from build123d import *

# Parameters (mm, degrees)
F1_DEPTH = 1.5875


with BuildPart() as f1:
    # F0 (on Top) → F1 (new body)
    with BuildSketch(Plane.XY):
        with BuildLine():
            ThreePointArc((0, 3.81), (2.694077, 2.694077), (3.81, 0))
            Line((3.81, 0), (59.69, 0))
            Line((59.69, 0), (59.69, 3.175))
            Line((59.69, 3.175), (66.04, 3.175))
            Line((66.04, 3.175), (66.04, 0))
            Line((66.04, 0), (74.93, 0))
            ThreePointArc((74.93, 0), (76.045923, 2.694077), (78.74, 3.81))
            Line((78.74, 3.81), (78.74, 31.75))
            Line((78.74, 31.75), (75.565, 31.75))
            Line((75.565, 31.75), (75.565, 34.925))
            Line((75.565, 34.925), (78.74, 34.925))
            Line((78.74, 34.925), (78.74, 62.23))
            ThreePointArc((78.74, 62.23), (76.045923, 63.345923), (74.93, 66.04))
            Line((74.93, 66.04), (3.81, 66.04))
            ThreePointArc((3.81, 66.04), (2.694077, 63.345923), (0, 62.23))
            Line((0, 62.23), (0, 3.81))
        make_face()
    extrude(amount=F1_DEPTH)


solid = f1.part
Can you work these out from the model? Positions are in its coordinate system, mm. A direction names the side the tool comes from. Coordinates: 2 decimals unless noted, no trailing zeros. Answer as CSV lines item,"result".
(1) If we mould it in two halves opening along X, with no side actions, what happens to faces 1 (the flat face through (31, 0, 1)), 2 (the flat face through (63, 3.175, 1)), 3 (the flat face through (59.69, 2, 1)), 4 (the flat face through (78.74, 18, 1))? For each: released by +X, released by -X, zero draft, split by the parting line, or undercut.
Geometry check:
face 1,"zero draft"
face 2,"undercut"
face 3,"undercut"
face 4,"released by +X"
(2) Please list where this line runs through material, in increasing order: L1, parallel to Y at x = 61, z = 1.3 (3 decimals).
Geometry check:
L1,"3.175 to 66.04"
(3) I'm going to push flat-ended pins straight in: pin 1 (0.8 mm diameter, centred on y = 32.5, z = 1, fed in from +X) (3 decimals); pin 2 (0.8 mm diameter, centred on y = 2.5, z = 1, fed in from -X); pin 3 (0.5 mm diameter, centred on y = 1.5, z = 1, fed in from +X). Where does each tip first touch, or does it pass through?
Geometry check:
pin 1,"x = 75.565"
pin 2,"x = 2.47"
pin 3,"x = 75.36"
(4) On a 3-axis mill with a long thin cutter (end or side, diameter ignored), from which of +Z, -Z, +X, -X, +Y, -Y can I reach the whole of each face in a straight line? I mean faces 5 (the flat face through (77, 34.925, 1)), 6 (the flat face through (66.04, 2, 1)), 7 (the cylindrical face through (76.016, 2.664, 0.783)). Say none if no direction works.
Geometry check:
face 5,"+Z, -Z, +X"
face 6,"+Z, -Z, -Y"
face 7,"+Z, -Z, +X, -Y"
